Could you check a few things on this model? Use its own coordinates, in mm. Give positions to 0.01 mm unless a question says otherwise; leave off trailing zeros. Write each loop counter-clockwise with the first axis right and the second up, starting at its lowest first coordinate (ties: lowest second). Pieces come first, ordered by that corner, then holes. Notation, with made-up numbers: (66.25, 53) - (80.25, 53) arc R23 ccw to (80.25, 80) - close; hole circle Ø7 at (-15, 17.25). An arc over 180 degrees is marked (long way). Answer as CSV lines item,"result". Start each with the question number.
Q1. Imagine slicing it at C-C on y = 1. List the corners of the cut face in (x, z) for me.
Q2. Imagine slicing it at D-D on z = 19. List the corners of the cut face in (x, y) for me (3 decimals), and give its area (3 significant figures).
Q3. Will these pins go through, and if not, where does the flat tip stop? pin 1 Ø5 at (x, z) = (-14, 19) entering from +Y; pin 2 Ø4 at (x, z) = (54, 19) entering from +Y.
Q4. Imagine slicing it at B-B on x = -14. List the corners of the cut face in (y, z) for me (3 decimals).
Q5. Imagine slicing it at A-A on z = -6. List the corners of the cut face in (x, y) for me, and give its area (3 significant figures).
Q6. If I drill on line 1 along X through (y, z) = (4.7, -19); line 2 along Z through (x, y) = (-14, 4.35); line 3 along X through (y, z) = (0.25, -8), over which ranges is the centre line in solid material (lowest first)?
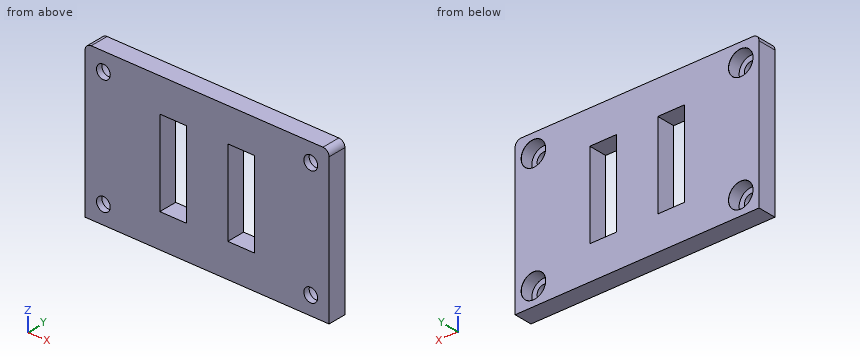
```python
from build123d import *

# Parameters (mm, degrees)
SKETCH2_W                     = 40
SKETCH2_H                     = 50
SKETCH2_W_2                   = 8.7
SKETCH2_H_2                   = 28
BOSS_EXTRUDE1_DEPTH           = 6
CBORE_FOR_M4_SHCS2_AT_2_COUNT = 2
CBORE_FOR_M4_SHCS2_AT_2_PITCH = 38
FILLET1_R                     = 2


with BuildPart() as part:
    # Sketch2 → Boss-Extrude1 (new body)
    with BuildSketch(Plane(origin=(0, 0, 0), x_dir=(1, 0, 0), z_dir=(0, 1, 0))):
        Rectangle(SKETCH2_W, SKETCH2_H)
        with Locations((8.85, 0)):
            Rectangle(SKETCH2_W_2, SKETCH2_H_2, mode=Mode.SUBTRACT)
    boss_extrude1 = extrude(amount=BOSS_EXTRUDE1_DEPTH)

    # Sketch4 → CBORE for M4 SHCS2 (revolve, cut)
    with BuildSketch(Plane(origin=(-14, 6, 19), x_dir=(0, 0, 1), z_dir=(1, 0, 0))):
        Polygon((0, 0), (0, 6), (2.25, 6), (2.25, 4), (4, 4), (4, 0.025), (4.025, 0), align=None)
    cbore_for_m4_shcs2 = revolve(axis=Axis((-14, 12.35, 19), (0, -1, 0)), mode=Mode.SUBTRACT)

    # CBORE for M4 SHCS2 at 2: CBORE for M4 SHCS2 ×2
    with Locations(*[(0, 0, -i * CBORE_FOR_M4_SHCS2_AT_2_PITCH) for i in range(1, CBORE_FOR_M4_SHCS2_AT_2_COUNT)]):
        add(cbore_for_m4_shcs2, mode=Mode.SUBTRACT)

    # Mirror1: Boss-Extrude1, CBORE for M4 SHCS2 across plane
    add(boss_extrude1.mirror(Plane(origin=(20, 0, 0), x_dir=(0, 0, 1), z_dir=(1, 0, 0))))
    add(cbore_for_m4_shcs2.mirror(Plane(origin=(20, 0, 0), x_dir=(0, 0, 1), z_dir=(1, 0, 0))), mode=Mode.SUBTRACT)

    # Mirror1 copy 1 sketch → Mirror1 copy 1 (revolve, cut)
    with BuildSketch(Plane(origin=(54, 6, -19), x_dir=(0, 0, 1), z_dir=(-1, 0, 0))):
        Polygon((0, 0), (0, -6), (2.25, -6), (2.25, -4), (4, -4), (4, -0.025), (4.025, 0), align=None)
    revolve(axis=Axis((54, 12.35, -19), (0, 1, 0)), mode=Mode.SUBTRACT)

    # Fillet1
    fillet1_edges = [part.edges().sort_by_distance(p)[0] for p in [
        (60, 3, 25),
        (-20, 3, 25),
    ]]
    fillet(fillet1_edges, radius=FILLET1_R)


solid = part.part
```
Conclusion:
1,outline,"(-20, -25) - (60, -25) - (60, 23) arc R2 ccw to (58, 25) - (-18, 25) arc R2 ccw to (-20, 23) - close; hole circle Ø4.5 at (-14, -19); hole circle Ø4.5 at (-14, 19); hole (4.5, -14) - (13.2, -14) - (13.2, 14) - (4.5, 14) - close; hole (26.8, -14) - (35.5, -14) - (35.5, 14) - (26.8, 14) - close; hole circle Ø4.5 at (54, -19); hole circle Ø4.5 at (54, 19)"
2,outline,"(-20, 0) - (-16.25, 0) - (-16.25, 2) - (-18, 2) - (-18, 5.975) - (-18.025, 6) - (-20, 6) - close; (-11.75, 0) - (51.75, 0) - (51.75, 2) - (50, 2) - (50, 5.975) - (49.975, 6) - (-9.975, 6) - (-10, 5.975) - (-10, 2) - (-11.75, 2) - close; (56.25, 0) - (60, 0) - (60, 6) - (58.025, 6) - (58, 5.975) - (58, 2) - (56.25, 2) - close"
2,area,"398 mm^2"
3,pin 1,"y = 2"
3,pin 2,"through"
4,outline,"(0, -25) - (6, -25) - (6, -23.025) - (5.975, -23) - (2, -23) - (2, -21.25) - (0, -21.25) - close; (0, -16.75) - (2, -16.75) - (2, -15) - (5.975, -15) - (6, -14.975) - (6, 14.975) - (5.975, 15) - (2, 15) - (2, 16.75) - (0, 16.75) - close; (0, 21.25) - (2, 21.25) - (2, 23) - (5.975, 23) - (6, 23.025) - (6, 25) - (0, 25) - close"
5,outline,"(-20, 0) - (4.5, 0) - (4.5, 6) - (-20, 6) - close; (13.2, 0) - (26.8, 0) - (26.8, 6) - (13.2, 6) - close; (35.5, 0) - (60, 0) - (60, 6) - (35.5, 6) - close"
5,area,"376 mm^2"
6,line 1,"-20 to -18, -10 to 50, 58 to 60"
6,line 2,"-25 to -23, -15 to 15, 23 to 25"
6,line 3,"-20 to 4.5, 13.2 to 26.8, 35.5 to 60"
